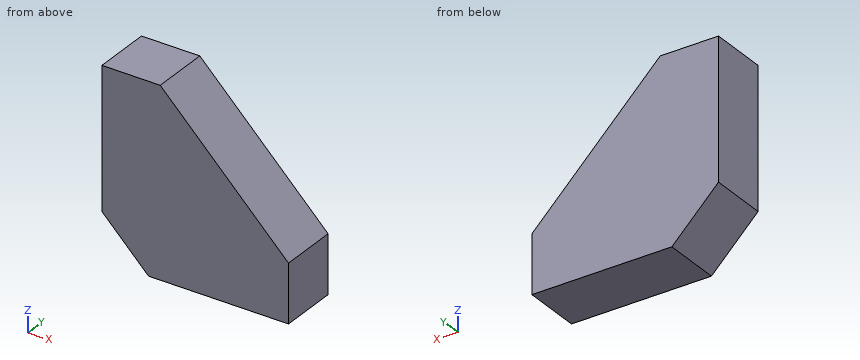
```python
from build123d import *

# Parameters (mm, degrees)
F1_DEPTH = 12.5


with BuildPart() as f1:
    # F0 (on Front) → F1 (new body, symmetric)
    with BuildSketch(Plane.XZ):
        Polygon((2450, 20), (2470, 0), (2530, 0), (2530, 25), (2475, 80), (2450, 80), align=None)
    extrude(amount=F1_DEPTH, both=True)


with BuildPart() as f2_1:
    # F2: copy of F1
    add(f1.part)


solid = f1.part
```
Source: CAD feature listing. Evaluate the final solid. Frame: model axes, mm. Round coordinates to 2 decimals unless told otherwise and drop trailing zeros. Write each loop counter-clockwise with the first axis right and the second up, starting at its lowest first coordinate (ties: lowest second). Pieces come first, ordered by that corner, then holes. Notation, with made-up numbers: M -21,73.25 L 18,73.25 A25 ccw 18,89.25 Z; hole C 37.25,66.5 d6. An arc over 180 degrees is marked long. Answer as a JSON object with one key per item and string values. Group by question number.
(1) Section query A-A on y = -10.5. Output: boundary loops of the cut face in (x, z).
(2) Section query C-C on z = 65. Output: boundary loops of the cut face in (x, y), then the cut area to 3 significant figures.
(3) Ray query, line 1 (Z direction, x = 2500.5, y = 5.5); line 2 (Z direction, x = 2515, y = -10.5); line 3 (X direction, y = -7, z = 5). Return the intervals inside material, ascending. Write a range as [from, to].
(4) Section query B-B on x = 2523.5. Output: boundary loops of the cut face in (y, z).
(5) First-contact query: pin 1 (5 mm diameter, centred on y = 5.5, z = 45, fed in from +X); pin 2 (1.5 mm diameter, centred on y = 8, z = 47.5, fed in from +X); pin 3 (5 mm diameter, centred on y = 2, z = 13, fed in from -X). Flat tips, straight axial feed; report the tip coordinate or a pass-through.
Computed values:
{
 "1": {"outline": "M 2450,20 L 2470,0 L 2530,0 L 2530,25 L 2475,80 L 2450,80 Z"},
 "2": {"outline": "M 2450,-12.5 L 2490,-12.5 L 2490,12.5 L 2450,12.5 Z", "area": "1,000 mm^2"},
 "3": {"line 1": "[0, 54.5]", "line 2": "[0, 40]", "line 3": "[2465, 2530]"},
 "4": {"outline": "M -12.5,0 L 12.5,0 L 12.5,31.5 L -12.5,31.5 Z"},
 "5": {"pin 1": "x = 2512.5", "pin 2": "x = 2508.25", "pin 3": "x = 2454.5"}
}
